For this review, take the finished solid that the model builds, in its own axes (mm). A direction names the side the tool comes from. Give positions to 0.01 mm unless a question says otherwise; leave off trailing zeros. Write each loop counter-clockwise with the first axis right and the second up, starting at its lowest first coordinate (ties: lowest second). Pieces come first, ordered by that corner, then holes. Notation, with made-up numbers: M 7.5,9 L 13.5,9 A11 cw 13.5,30 Z; hole C -13,14.25 d7. An arc over 180 degrees is marked long. Write item = value, one per line.
```python
from build123d import *

# Parameters (mm, degrees)
SKETCH1_W                                           = 1270
SKETCH1_H                                           = 1270
SKETCH1_R                                           = 63.5
BOSS_EXTRUDE1_DEPTH                                 = 254
CBORE_FOR_00_BINDING_HEAD_MACHINE_SCREW_D           = 76.2
CBORE_FOR_00_BINDING_HEAD_MACHINE_SCREW_CBORE_D     = 127
CBORE_FOR_00_BINDING_HEAD_MACHINE_SCREW_CBORE_DEPTH = 76.2


with BuildPart() as part:
    # Sketch1 → Boss-Extrude1 (new body)
    with BuildSketch(Plane(origin=(0, 0, 0), x_dir=(1, 0, 0), z_dir=(0, 1, 0))):
        Rectangle(SKETCH1_W, SKETCH1_H)
        with Locations(Location((-381, -381, 0), (0, 0, 270))):
            Circle(SKETCH1_R, mode=Mode.SUBTRACT)
        with Locations(Location((-535.427409328, 60.328180312, 0), (0, 0, 270))):
            Circle(SKETCH1_R, mode=Mode.SUBTRACT)
        with Locations(Location((-286.667058704, 456.228010379, 0), (0, 0, 270))):
            Circle(SKETCH1_R, mode=Mode.SUBTRACT)
        with Locations(Location((177.959434067, 508.578843275, 0), (0, 0, 270))):
            Circle(SKETCH1_R, mode=Mode.SUBTRACT)
        with Locations(Location((508.578843275, 177.959434067, 0), (0, 0, 270))):
            Circle(SKETCH1_R, mode=Mode.SUBTRACT)
        with Locations(Location((456.228010379, -286.667058704, 0), (0, 0, 270))):
            Circle(SKETCH1_R, mode=Mode.SUBTRACT)
        with Locations(Location((60.328180312, -535.427409328, 0), (0, 0, 270))):
            Circle(SKETCH1_R, mode=Mode.SUBTRACT)
    extrude(amount=BOSS_EXTRUDE1_DEPTH)

    # CBORE for #00 Binding Head Machine Screw1 (through all)
    with Locations(Plane(origin=(0, 254, 0), x_dir=(1, 0, 0), z_dir=(0, 1, 0))):
        with Locations((0, 0)):
            CounterBoreHole(CBORE_FOR_00_BINDING_HEAD_MACHINE_SCREW_D / 2, CBORE_FOR_00_BINDING_HEAD_MACHINE_SCREW_CBORE_D / 2, CBORE_FOR_00_BINDING_HEAD_MACHINE_SCREW_CBORE_DEPTH)


solid = part.part
```
1. For line 1 along Z through (x, y) = (514, 191); line 2 along X through (y, z) = (115, 341); line 3 along Z through (x, y) = (461, 176), list the stretches that pass through material, from the lowest coordinate up. Write a range as from..to.
Responses:
line_1 = -635..-241.23, -114.69..260.31, 313.02..635
line_2 = -635..-430.32, -331.68..423.36, 489.09..635
line_3 = -635..-220.01, -135.91..223.35, 349.99..635
2. We need section C-C, the plane y = 127.5. Count the separate pieces of the cut face and the enclosed holes in it, then the cut area to 3 significant figures.
Responses:
separate_pieces = 1
enclosed_holes = 8
area = 1,520,000 mm2
3. We need section A-A, the plane z = 381. Write out the cut boundary in (x, y), then the cut area to 3 significant figures.
Responses:
outline = M -635,0 L -444.5,0 L -444.5,254 L -635,254 Z; M -317.5,0 L 635,0 L 635,254 L -317.5,254 Z
area = 290,000 mm2
4. Machinability: for faces 5 (the face through (-13.77, 216.43, 61.99)), 6 (the face through (-437.335, 125.222, 410.301)), which of the approach directions +Z, -Z, +X, -X, +Y, -Y give a long, thin tool a straight path to every point of the face, cutting with its end or side? Answer none if there is none.
Responses:
face_5 = +Y
face_6 = +Y, -Y
5. The part is to be moulded in two halves that separate along X. For faces 1 (the face through (-150, 254, -9)), 2 (the face through (231.5, 125.22, -474.44)), 3 (the face through (-635, 125, 9)), 4 (the face through (-267.59, 125.22, -395.66)), say which applies: +X half, -X half, draft (parallel to the pull), parting line (faces both ways), or undercut.
Responses:
face_1 = draft
face_2 = undercut
face_3 = -X half
face_4 = undercut
6. We need section B-B, the plane x = -381. Write out the cut boundary in (y, z).
Responses:
outline = M 0,-635 L 254,-635 L 254,317.5 L 0,317.5 Z; M 0,444.5 L 254,444.5 L 254,635 L 0,635 Z
